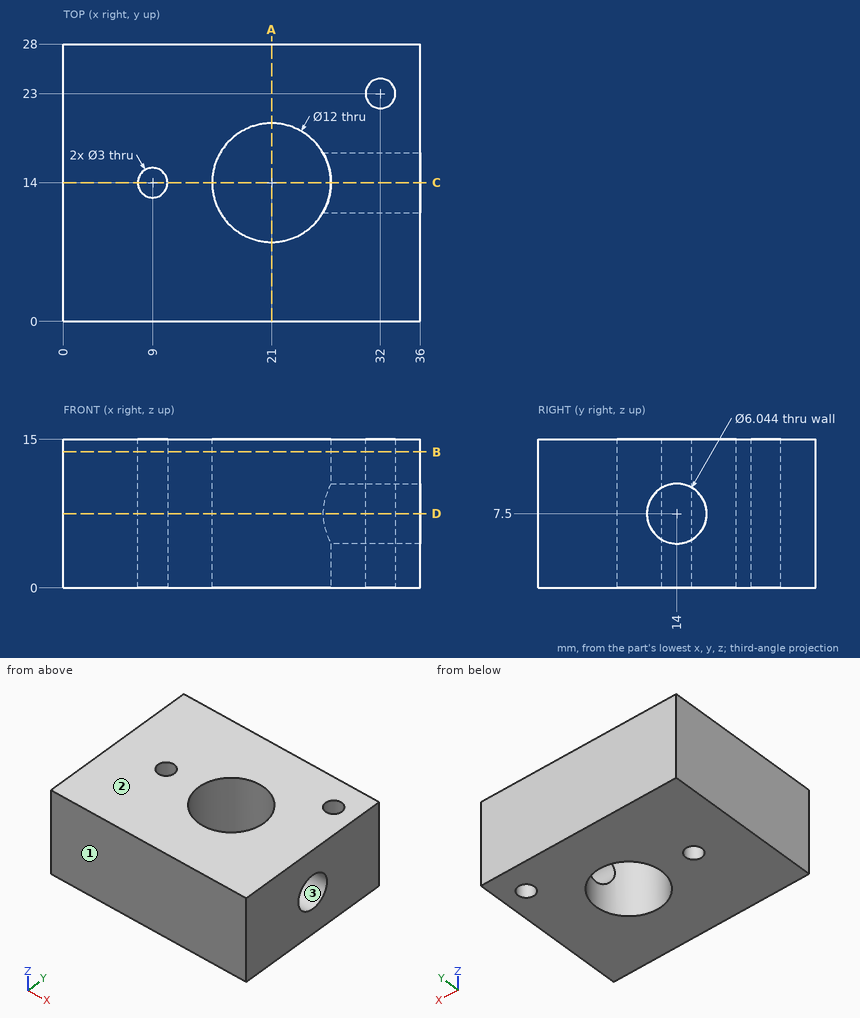
Print and shaded views of the part. All mm, measured from the part's lowest x, y and z. Coordinates: 2 decimals unless noted, no trailing zeros. Write each loop counter-clockwise with the first axis right and the second up, starting at its lowest first coordinate (ties: lowest second). Pieces come first, ordered by that corner, then holes. Notation, with made-up numbers: (25, 43) - (33, 43) arc R23 ccw to (33, 54) - close; hole circle Ø10 at (76.25, -5.75). An arc over 180 degrees is marked (long way). One line per question, with ' | ' between items. Start each with the question number.
Q1. Drill centre lines: line 1 (Y direction, x = 21, z = 6); line 2 (Y direction, x = 9, z = 12); line 3 (X direction, y = 10.75, z = 6). Where is each one in solid material? Low to high. Write a range as [from, to].
Q2. Cut at B-B, the plane z = 13.75. List the corners of the cut face in (x, y), then the cut area to 3 significant figures.
Q3. Cut at C-C, the plane y = 14. List the corners of the cut face in (x, z).
Q4. Cut at D-D, the plane z = 7.5. List the corners of the cut face in (x, y).
Q5. Pin check, flat tips, straight feed: pin 1 (3.5 mm diameter, centred on y = 14, z = 7.5, fed in from +X); pin 2 (1.8 mm diameter, centred on x = 9, y = 14, fed in from -Z). Stop position of each tip, or through.
Q6. Cut at A-A, the plane x = 21. List the corners of the cut face in (y, z), then the cut area to 3 significant figures.
Q7. Pull direction Z, two halves, no side cores. Call the marked faces 1, 2 and 3: pulls with the +Z half, pulls with the -Z half, needs draft (parallel to the pull), parting line crosses it, or undercut.
Answer below:
1) line 1: [0, 8], [20, 28] | line 2: [0, 12.5], [15.5, 28] | line 3: [0, 15.96], [26.04, 36]
2) outline: (0, 0) - (36, 0) - (36, 28) - (0, 28) - close; hole circle Ø3 at (9, 14); hole circle Ø12 at (21, 14); hole circle Ø3 at (32, 23) | area: 881 mm^2
3) outline: (0, 0) - (7.5, 0) - (7.5, 15) - (0, 15) - close; (10.5, 0) - (15, 0) - (15, 15) - (10.5, 15) - close; (27, 0) - (36, 0) - (36, 4.48) - (27, 4.48) - close; (27, 10.52) - (36, 10.52) - (36, 15) - (27, 15) - close
4) outline: (0, 0) - (36, 0) - (36, 10.98) - (26.18, 10.98) arc R6 cw (long way) to (26.18, 17.02) - (36, 17.02) - (36, 28) - (0, 28) - close; hole circle Ø3 at (9, 14); hole circle Ø3 at (32, 23)
5) pin 1: x = 15.26 | pin 2: through
6) outline: (0, 0) - (8, 0) - (8, 15) - (0, 15) - close; (20, 0) - (28, 0) - (28, 15) - (20, 15) - close | area: 240 mm^2
7) face 1: needs draft | face 2: pulls with the +Z half | face 3: undercut
